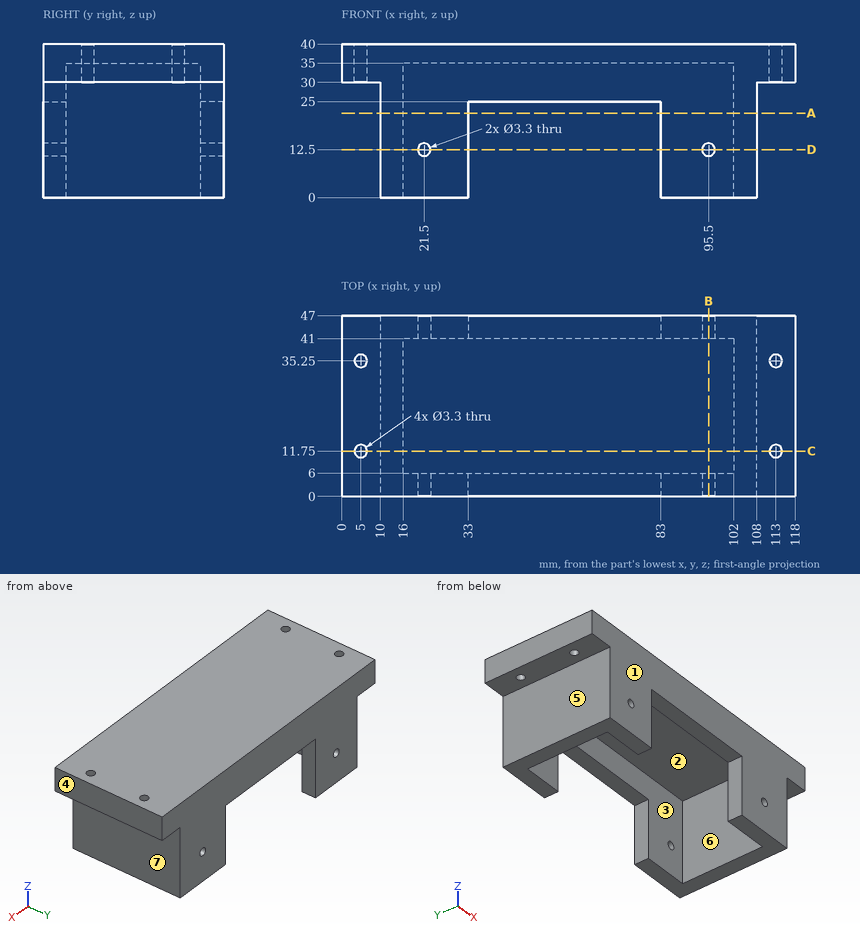
The drawing under review shows one solid part. Ordinate dimensions are in mm from its lowest x, y, z. A direction names the side the tool comes from. Round coordinates to 2 decimals unless told otherwise and drop trailing zeros. Order: outer loops, then holes, each group sorted by start corner. A loop starts at its lowest first (then second) coordinate and runs counter-clockwise, first axis right, second up. Notation, with made-up numbers: (-7.75, -32) -> (49.25, -32) arc R27 cw to (49.25, -10) -> close; hole circle Ø6 at (89, 63.25). An arc over 180 degrees is marked (long way). Return JSON: item names as keys, results as strings.
1. Take a section at C-C (y = 11.75). Write out the cut boundary in (x, z), then the cut area to 3 significant figures.
Answer block:
{"outline": "(0, 30) -> (3.35, 30) -> (3.35, 40) -> (0, 40) -> close; (6.65, 30) -> (10, 30) -> (10, 0) -> (16, 0) -> (16, 35) -> (102, 35) -> (102, 0) -> (108, 0) -> (108, 30) -> (111.35, 30) -> (111.35, 40) -> (6.65, 40) -> close; (114.65, 30) -> (118, 30) -> (118, 40) -> (114.65, 40) -> close", "area": "1,040 mm²"}
2. The part is to be moulded in two halves that separate along X. For the marked faces 1, 2, 3 and 4, say which applies: +X half, -X half, draft (parallel to the pull), parting line (faces both ways), or undercut.
Answer block:
{"face 1": "draft", "face 2": "undercut", "face 3": "undercut", "face 4": "+X half"}
3. Take a section at B-B (x = 95.5). Write out the cut boundary in (y, z), then the cut area to 3 significant figures.
Answer block:
{"outline": "(0, 0) -> (6, 0) -> (6, 10.85) -> (0, 10.85) -> close; (0, 14.15) -> (6, 14.15) -> (6, 35) -> (41, 35) -> (41, 14.15) -> (47, 14.15) -> (47, 40) -> (0, 40) -> close; (41, 0) -> (47, 0) -> (47, 10.85) -> (41, 10.85) -> close", "area": "615 mm²"}
4. Take a section at D-D (z = 12.5). State how many separate pieces and enclosed holes the cut face has, then the cut area to 3 significant figures.
Answer block:
{"separate pieces": "6", "enclosed holes": "0", "area": "917 mm²"}
5. Take a section at A-A (z = 22). Write out the cut boundary in (x, y), then the cut area to 3 significant figures.
Answer block:
{"outline": "(10, 0) -> (33, 0) -> (33, 6) -> (16, 6) -> (16, 41) -> (33, 41) -> (33, 47) -> (10, 47) -> close; (83, 0) -> (108, 0) -> (108, 47) -> (83, 47) -> (83, 41) -> (102, 41) -> (102, 6) -> (83, 6) -> close", "area": "996 mm²"}
6. Insertion check: P1, Ø1.5, axis at x = 20.5, y = 29, coming from the -Z side; P2, Ø11, axis at x = 115, y = 15, coming from the -Z side; P3, Ø3, axis at y = 38, z = 21, coming from the +X side. Each pin has a flat end and moves straight along its axis. Give the tip position at first contact, or say it passes through.
Answer block:
{"P1": "stops at z = 35", "P2": "stops at z = 30", "P3": "stops at x = 108"}
7. For the marked faces 5, 6 and 7, list the 3-axis set-ups (+Z, -Z, +X, -X, +Y, -Y) from which the entire face can be reached by the end or side of a thin tool; tool diameter is ignored.
Answer block:
{"face 5": "-Z, -X, +Y, -Y", "face 6": "-Z", "face 7": "-Z, +X, +Y, -Y"}
8. For L1, parallel to X at y = 1.9, z = 12.5; L2, parallel to Y at x = 5, z = 36.5; L3, parallel to X at y = 16, z = 17, list the stretches that pass through material, from the lowest coordinate up. Write a range as [from, to].
Answer block:
{"L1": "x = [10, 19.85], [23.15, 33], [83, 93.85], [97.15, 108]", "L2": "y = [0, 10.1], [13.4, 33.6], [36.9, 47]", "L3": "x = [10, 16], [102, 108]"}
